Drawing for the job (mm, zero at the part's lowest x, y, z). A direction names the side the tool comes from. Coordinates: 2 decimals unless noted, no trailing zeros. Loops run counter-clockwise (first coordinate to the right, second up) from the corner with the lowest first, then second, coordinate; pieces in that order, holes last.
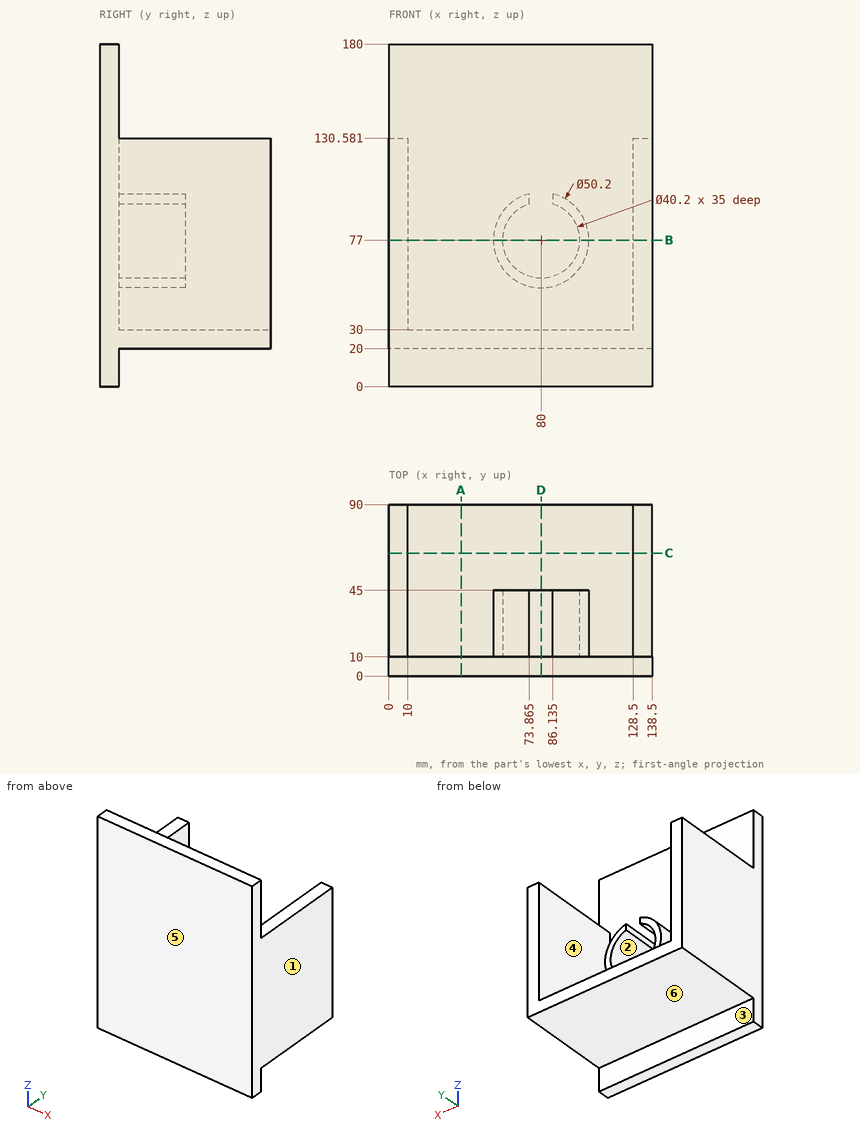
Q1. Tool access for the marked faces 4, 5 and 6: list every direction of +Z, -Z, +X, -X, +Y, -Y with a clear straight run to the whole face (end or side of a thin tool).
Q2. Drop flat-ended pins along their axis: P1, Ø8, axis at x = 69, y = 39, coming from the -Z side; P2, Ø4, axis at x = 36, z = 34.5, coming from the +Y side; P3, Ø5, axis at x = 131.5, y = 62, coming from the +Z side. Give the stop position or say it passes through.
Q3. Saw through at C-C (y = 64.5). List the corners of the cut face in (x, z), plus the area to 3 significant figures.
Q4. Saw through at B-B (z = 77). List the corners of the cut face in (x, y), plus the area to 4 significant figures.
Q5. Mould opens along X. For the marked faces 1, 2 and 3 say: released by +X, released by -X, zero draft, split by the parting line, or undercut.
Q6. Saw through at A-A (x = 38). List the corners of the cut face in (y, z), plus the area to 3 significant figures.
Q7. Probe line 1 (X direction, y = 29, z = 77); line 2 (X direction, y = 69, z = 121.5); line 3 (Z direction, x = 80, y = 24.5). List the from-to ranges inside material, lowest first.
Q8. Saw through at D-D (x = 80). List the corners of the cut face in (y, z).
Checked values:
1. face 4: +Z, +Y
1. face 5: +Z, -Z, +X, -X, -Y
1. face 6: -Z, +X, -X, +Y
2. P1: stops at z = 20
2. P2: stops at y = 10
2. P3: stops at z = 130.58
3. outline: (0, 20) - (138.5, 20) - (138.5, 130.58) - (128.5, 130.58) - (128.5, 30) - (10, 30) - (10, 130.58) - (0, 130.58) - close
3. area: 3,400 mm2
4. outline: (0, 0) - (138.5, 0) - (138.5, 90) - (128.5, 90) - (128.5, 10) - (105.1, 10) - (105.1, 45) - (100.1, 45) - (100.1, 10) - (59.9, 10) - (59.9, 45) - (54.9, 45) - (54.9, 10) - (10, 10) - (10, 90) - (0, 90) - close
4. area: 3,335 mm2
5. face 1: released by +X
5. face 2: undercut
5. face 3: zero draft
6. outline: (0, 0) - (10, 0) - (10, 20) - (90, 20) - (90, 30) - (10, 30) - (10, 180) - (0, 180) - close
6. area: 2,600 mm2
7. line 1: x = 0 to 10, 54.9 to 59.9, 100.1 to 105.1, 128.5 to 138.5
7. line 2: x = 0 to 10, 128.5 to 138.5
7. line 3: z = 20 to 30, 51.9 to 56.9
8. outline: (0, 0) - (10, 0) - (10, 20) - (90, 20) - (90, 30) - (10, 30) - (10, 51.9) - (45, 51.9) - (45, 56.9) - (10, 56.9) - (10, 180) - (0, 180) - close
